from build123d import *

# Parameters (mm, degrees)
BOSS_EXTRUDE1_DEPTH = 45.5
CUT_EXTRUDE1_REACH  = 58.087
SKETCH3_W           = 51
SKETCH3_H           = 7.5
SKETCH3_W_2         = 40
SKETCH3_H_2         = 6
BOSS_EXTRUDE2_DEPTH = 10
CUT_EXTRUDE3_DEPTH  = 93.863842547


with BuildPart() as part:
    # Sketch2 → Boss-Extrude1 (new, symmetric)
    with BuildSketch(Plane(origin=(0, 0, 0), x_dir=(0, 0, -1), z_dir=(1, 0, 0))):
        Polygon((-13.625543001, 3.368080573), (-15.780269904, 9.288144084), (-8.732575248, 11.853295159), (-16.806330334, 12.107221947), (-20.565100817, 10.739141373), (-17.384313485, 2), (-16.656373016, 0), (22.718204566, 0), (17.384313485, 14.654745303), (14.203526152, 23.393886676), (9.891430857, 21.824412342), (9.591430857, 18.522687954), (11.470816098, 19.206728241), (13.625543001, 13.28666473), align=None)
    extrude(amount=BOSS_EXTRUDE1_DEPTH, both=True)

    # Sketch3 → Cut-Extrude1 (cut, up to next)
    with BuildSketch(Plane(origin=(0, 16.092396472, 5.857153314), x_dir=(1, 0, 0), z_dir=(0, 0.9396926207859102, 0.34202014332566394)), mode=Mode.PRIVATE) as cut_extrude1_sk1:
        with Locations((0, -7.901870812)):
            Rectangle(SKETCH3_W, SKETCH3_H)
    cut_extrude1_tool1 = extrude(cut_extrude1_sk1.sketch, amount=-CUT_EXTRUDE1_REACH, mode=Mode.PRIVATE) & part.part
    # Sketch3 → Cut-Extrude1 (cut, up to next)
    with BuildSketch(Plane(origin=(0, 16.092396472, 5.857153314), x_dir=(1, 0, 0), z_dir=(0, 0.9396926207859102, 0.34202014332566394)), mode=Mode.PRIVATE) as cut_extrude1_sk2:
        with Locations((0, 18.348129188)):
            Rectangle(SKETCH3_W_2, SKETCH3_H_2)
    cut_extrude1_tool2 = extrude(cut_extrude1_sk2.sketch, amount=-CUT_EXTRUDE1_REACH, mode=Mode.PRIVATE) & part.part
    add(cut_extrude1_tool1.solids().sort_by_distance((0, 13.389797, 13.282483))[0], mode=Mode.SUBTRACT)
    add(cut_extrude1_tool2.solids().sort_by_distance((0, 22.367826, -11.384448))[0], mode=Mode.SUBTRACT)

    # Sketch4 → Boss-Extrude2 (add)
    with BuildSketch(Plane.XZ):
        with BuildLine():
            Line((41.45, 4.894084225), (41.45, -10.955915775))
            ThreePointArc((41.45, -10.955915775), (39.775, -12.630915775), (38.1, -10.955915775))
            Line((38.1, -10.955915775), (38.1, 4.894084225))
            ThreePointArc((38.1, 4.894084225), (39.775, 6.569084225), (41.45, 4.894084225))
        make_face()
        with BuildLine():
            Line((-41.45, 4.894084225), (-41.45, -10.955915775))
            ThreePointArc((-41.45, -10.955915775), (-39.775, -12.630915775), (-38.1, -10.955915775))
            Line((-38.1, -10.955915775), (-38.1, 4.894084225))
            ThreePointArc((-38.1, 4.894084225), (-39.775, 6.569084225), (-41.45, 4.894084225))
        make_face()
    extrude(amount=BOSS_EXTRUDE2_DEPTH)

    # Sketch5 → Cut-Extrude3 (cut, through all)
    with BuildSketch(Plane(origin=(41.45, 0, 0), x_dir=(0, 0, -1), z_dir=(1, 0, 0))):
        Polygon((-6.569084225, -1.827958291), (10.955915775, -10), (-6.569084225, -10), align=None)
    extrude(amount=-CUT_EXTRUDE3_DEPTH, mode=Mode.SUBTRACT)


solid = part.part
Check sheet for the modelled part. Datum: model origin and axes. Units: mm. A direction names the side the tool comes from. Round coordinates to 2 decimals unless told otherwise and drop trailing zeros. Order: outer loops, then holes, each group sorted by start corner. A loop starts at its lowest first (then second) coordinate and runs counter-clockwise, first axis right, second up. Notation, with made-up numbers: M -22.75,12.25 L -14.75,12.25 A21 cw -14.75,42.25 Z; hole C 34,39.5 d11. An arc over 180 degrees is marked long. One line per item, written item: value. Start each with the question number.
1. Scan lines: line 1 along X through (y, z) = (-3.5, -10); line 2 along X through (y, z) = (3.5, -20); line 3 along Y through (x, z) = (-34, 16). Record each from-to range of solid material in increasing order.
2. Section check D-D on x = 21. Enter the section's corners in (y, z), and give its area (3 significant figures).
3. Section check A-A on x = -13.5. Enter the section's corners in (y, z), and give its area (3 significant figures).
4. Access from +Z, -Z, +X, -X, +Y, -Y to the whole of each face (thin tool, end or side, straight path). Record for faces 4 (the cylindrical face through (-39.81, -4.93, -12.63)), 5 (the flat face through (-0.28, 6.39, -14.008)), 6 (the cylindrical face through (39.74, -1, 6.57)), 7 (the flat face through (-38.1, -4, -5)).
5. Section check C-C on y = -6. Enter the section's corners in (x, z) (3 decimals).
6. Release check for a two-part mould opening along Z. For faces 1 (the flat face through (-20, 11, -16)), 2 (the flat face through (-25.5, 11, 14)), 3 (the flat face through (32.93, 22.62, -12.08)) record: released by +Z, released by -Z, zero draft, split by the parting line, or undercut.
7. Section check B-B on z = -20. Enter the section's corners in (x, y), and give its area (3 significant figures).
8. Gauge pin test, flat ends, axial feed: P1, Ø11, axis at y = -4, z = 1, coming from the -X side; P2, Ø10, axis at x = -23.5, z = -13.5, coming from the -Y side; P3, Ø10, axis at x = 3, z = -2, coming from the +Y side; P4, Ø12, axis at x = 26.5, y = 16.5, coming from the -Z side. Record the tip position at first contact, or that the pin passes through.
Results found:
1. line 1: -41.45 to -38.1, 38.1 to 41.45
1. line 2: -45.5 to -20, 20 to 45.5
1. line 3: 0 to 12.08
2. outline: M 0,-22.72 L 23.39,-14.2 L 21.82,-9.89 L 18.52,-9.59 L 19.21,-11.47 L 13.29,-13.63 L 3.37,13.63 L 12.11,16.81 L 10.74,20.57 L 0,16.66 Z
2. area: 406 mm^2
3. outline: M 0,-16.33 L 12.6,-11.75 L 3.37,13.63 L 12.11,16.81 L 10.74,20.57 L 0,16.66 Z
3. area: 278 mm^2
4. face 4: -Z, -Y
4. face 5: -Z, +Y
4. face 6: +Z, -Y
4. face 7: +Z, -Z, -Y
5. outline: M -41.45,-10.956 A1.675 ccw -38.1,-10.956 L -38.1,-2.378 L -41.45,-2.378 Z; M 38.1,-10.956 A1.675 ccw 41.45,-10.956 L 41.45,-2.378 L 38.1,-2.378 Z
6. face 1: zero draft
6. face 2: undercut
6. face 3: released by +Z
7. outline: M -45.5,0 L -20,0 L -20,7.47 L -45.5,7.47 Z; M 20,0 L 45.5,0 L 45.5,7.47 L 20,7.47 Z
7. area: 381 mm^2
8. P1: x = -45.5
8. P2: y = 0
8. P3: y = 10.88
8. P4: z = -18.9
